```python
from build123d import *

# Parameters (mm, degrees)
F0_W     = 6
F0_H     = 0.3
F1_DEPTH = 7
F2_W     = 76
F2_H     = 36
F3_DEPTH = 2
F4_R     = 2


# Not quite as in the source:
# - a feature names something its author has since deleted; it is built from what else it names


with BuildPart() as f1:
    # F0 (on Top) → F1 (new body)
    with BuildSketch(Plane.XY):
        Polygon((3.5, 0), (-3.5, 0), (-3.5, -65), (-23.5, -65), (-23.5, -70), (-17.5, -70), (-3.6, -70), (-3.6, -66.9), (3.6, -66.9), (3.6, -70), (17.5, -70), (23.5, -70), (23.5, -65), (3.5, -65), align=None)
        with Locations((-20.5, -70.15)):
            Rectangle(F0_W, F0_H)
        with Locations((20.5, -70.15)):
            Rectangle(F0_W, F0_H)
        Polygon((-40, 40), (-40, 0), (-3.5, 0), (3.5, 0), (40, 0), (40, 40), align=None)
    extrude(amount=F1_DEPTH)

    # F2 (on face) → F3 (cut)
    with BuildSketch(Plane.XY.offset(7)):
        with Locations((0, 20)):
            Rectangle(F2_W, F2_H)
    extrude(amount=-F3_DEPTH, mode=Mode.SUBTRACT)

    # F4
    f4_edges = [f1.edges().sort_by_distance(p)[0] for p in [
        (-3.5, 0, 3.5),
        (3.5, 0, 3.5),
        (3.5, -65, 3.5),
        (-3.5, -65, 3.5),
        (-23.5, -65, 3.5),
        (23.5, -65, 3.5),
        (-23.5, -70.3, 3.5),
        (23.5, -70.3, 3.5),
        (40, 0, 3.5),
        (-40, 0, 3.5),
    ]]
    fillet(f4_edges, radius=F4_R)


solid = f1.part
```
Check sheet for the modelled part. Datum: model origin and axes. Units: mm. A direction names the side the tool comes from. Round coordinates to 2 decimals unless told otherwise and drop trailing zeros. Loops run counter-clockwise (first coordinate to the right, second up) from the corner with the lowest first, then second, coordinate; pieces in that order, holes last. Notation, with made-up numbers: (64, 23) - (123, 23) arc R26 ccw to (123, 47) - close; hole circle Ø3 at (-37.5, 40). An arc over 180 degrees is marked (long way). Write item = value, one per line. Start each with the question number.
Q1. Section check C-C (x = -33). Record the boundary of the cut face in (y, z).
Q2. Section check A-A (x = -8.5). Record the boundary of the cut face in (y, z).
Q3. Access from +Z, -Z, +X, -X, +Y, -Y to the whole of each face (thin tool, end or side, straight path). Record for faces 4 (the face through (-22, 0, 3)), 5 (the face through (-40, 21, 3)), 6 (the face through (-1, 20, 5)), 7 (the face through (22, 0, 3)), 8 (the face through (3.6, -68, 3)).
Q4. Release check for a two-part mould opening along Y. For faces 1 (the face through (-1, 10, 0)), 2 (the face through (3.5, -33, 3)), 3 (the face through (19, -70.3, 3)) record: pulls with the +Y half, pulls with the -Y half, needs draft (parallel to the pull), parting line crosses it, or undercut.
Q5. Depth check by flat-ended pin: P1, Ø1, axis at y = -67.5, z = 3, coming from the -X side; P2, Ø3.5, axis at x = -29.5, z = 4, coming from the -Y side; P3, Ø2, axis at x = -16, z = 5.5, coming from the -Y side. Enter the tip coordinate at first touch or a pass-through.
Q6. Section check B-B (y = 10.5). Record the boundary of the cut face in (x, z), plus the area to 3 significant figures.
Q7. Thickness scan on L1, parallel to Y at x = -21.5, z = 6.5; L2, parallel to Y at x = 17, z = 4.5; L3, parallel to Y at x = -25, z = 6. Record the ranges inside material, lowest first.
Derived:
q1.outline = (0, 0) - (40, 0) - (40, 7) - (38, 7) - (38, 5) - (2, 5) - (2, 7) - (0, 7) - close
q2.outline = (-70, 0) - (-65, 0) - (-65, 7) - (-70, 7) - close; (0, 0) - (40, 0) - (40, 7) - (38, 7) - (38, 5) - (2, 5) - (2, 7) - (0, 7) - close
q3.face_4 = +Z, -Z, -X
q3.face_5 = +Z, -Z, -X, +Y, -Y
q3.face_6 = +Z
q3.face_7 = +Z, -Z, +X
q3.face_8 = +Z, -Z, -Y
q4.face_1 = needs draft
q4.face_2 = undercut
q4.face_3 = pulls with the -Y half
q5.P1 = -23.5
q5.P2 = 0
q5.P3 = -70
q6.outline = (-40, 0) - (40, 0) - (40, 7) - (38, 7) - (38, 5) - (-38, 5) - (-38, 7) - (-40, 7) - close
q6.area = 408 mm^2
q7.L1 = -70.3 to -65, 0 to 2, 38 to 40
q7.L2 = -70 to -65, 0 to 40
q7.L3 = 0 to 2, 38 to 40
